Check sheet for the modelled part. Datum: model origin and axes. Units: mm. A direction names the side the tool comes from. Coordinates: 2 decimals unless noted, no trailing zeros. Loops run counter-clockwise (first coordinate to the right, second up) from the corner with the lowest first, then second, coordinate; pieces in that order, holes last.
```python
from build123d import *

# Parameters (mm, degrees)
F0_W     = 23.4204549342
F0_H     = 2.8636362404
F3_R     = 5
F5_W     = 35.1818175986
F5_H     = 36.409093067
F6_DEPTH = 64


# Not quite as in the source:
# - a fillet or chamfer that OpenCascade refuses, or shapes differently, is made with other operations: its cross-section is extruded or revolved along the edge and cut away or added


with BuildPart() as f1:
    # F0 (on Top) → F1 (revolve)
    with BuildSketch(Plane.XY):
        Polygon((-23.4204549342, 28.6363661289), (-26.4886375517, 28.6363661289), (-26.4886375517, -20.4545464367), (-23.4204549342, -20.4545464367), (-23.4204549342, -17.5909101963), align=None)
        with Locations((-11.7102274671, -19.0227283165)):
            Rectangle(F0_W, F0_H)
    revolve(axis=Axis((0, -19.0227283165, 0), (0, 1, 0)))

    # F3
    f3_edges = [f1.edges().sort_by_distance(p)[0] for p in [
        (26.488638, -20.454546, 0),
    ]]
    fillet(f3_edges, radius=F3_R)

    # F4: fillet of radius 5 on 1 edges, made by hand

    # F4_s1 → F4_t2 (revolve, cut)
    with BuildSketch(Plane.XY):
        with BuildLine():
            ThreePointArc((-26.4886375517, 28.6363661289), (-24.2575781097, 26.7941920001), (-23.4204549342, 24.0246330924))
            Line((-23.4204549342, 24.0246330924), (-23.4204549342, 28.6363661289))
            Line((-23.4204549342, 28.6363661289), (-26.4886375517, 28.6363661289))
        make_face()
    revolve(axis=Axis((0, 28.6363661289, 0), (0, 1, 0)), mode=Mode.SUBTRACT)

    # F5 (on offset) → F6 (cut)
    with BuildSketch(Plane.YZ.offset(-26.45)):
        with Locations((7.4659097008, -1.0227272287)):
            Rectangle(F5_W, F5_H)
    extrude(amount=-F6_DEPTH, mode=Mode.SUBTRACT)


solid = f1.part
```
1) Section check A-A on z = 0. Enter the section's corners in (x, y) (3 decimals), plus the area to 3 significant figures.
Answer sheet:
outline: (-26.489, -15.455) arc R5 ccw to (-21.489, -20.455) - (21.489, -20.455) arc R5 ccw to (26.489, -15.455) - (26.489, 28.636) arc R5 ccw to (23.42, 24.025) - (23.42, -17.591) - (-23.42, -17.591) - (-23.42, 24.025) arc R5 ccw to (-26.489, 28.636) - (-26.489, 25.057) - (-26.45, 25.057) - (-26.45, -10.125) - (-26.489, -10.125) - close
area: 415 mm2
2) Section check C-C on y = 10. Enter the section's corners in (x, z).
Answer sheet:
outline: (-26.45, -1.43) arc R26.49 ccw (long way) to (-26.45, 1.43) - close; hole circle Ø46.84 at (0, 0)
3) Depth check by flat-ended pin: pin 1 (6 mm diameter, centred on y = 14, z = 14, fed in from +X); pin 2 (8 mm diameter, centred on y = -9, z = 6.5, fed in from -X); pin 3 (10 mm diameter, centred on y = 19.5, z = -14.5, fed in from -X). Enter the tip coordinate at first touch or a pass-through.
Answer sheet:
pin 1: stops at x = 24.1
pin 2: stops at x = -26.37
pin 3: stops at x = -24.73
4) Set-up check for faces 1 (the cylindrical face through (5.077, 3.508, -22.864)), 2 (the flat face through (0, -20.455, 0)): record each of +Z, -Z, +X, -X, +Y, -Y from which the full face is reachable in a straight line by a thin tool's end or side.
Answer sheet:
face 1: +Y
face 2: +Z, -Z, +X, -X, -Y
5) Mould release check, pull along X, two halves, no side actions. Record for faces 3 (the cylindrical face through (-25.265, 6.282, 7.956)), 4 (the flat face through (-26.45, 7, 0)), 5 (the flat face through (0, -17.591, 0)): +X half, -X half, draft (parallel to the pull), parting line (faces both ways), or undercut.
Answer sheet:
face 3: parting line
face 4: -X half
face 5: undercut
6) Section check B-B on x = 0. Enter the section's corners in (y, z), plus the area to 3 significant figures.
Answer sheet:
outline: (-20.45, -21.49) arc R5 ccw to (-15.45, -26.49) - (28.64, -26.49) arc R5 ccw to (24.02, -23.42) - (-17.59, -23.42) - (-17.59, 23.42) - (24.02, 23.42) arc R5 ccw to (28.64, 26.49) - (-15.45, 26.49) arc R5 ccw to (-20.45, 21.49) - close
area: 417 mm2
7) Scan lines: line 1 (Z direction, x = 0, y = 8); line 2 (Y direction, x = 16, z = -9); line 3 (Z direction, x = -9, y = 14). Record each from-to range of solid material in increasing order.
Answer sheet:
line 1: z = -26.49 to -23.42, 23.42 to 26.49
line 2: y = -20.45 to -17.59
line 3: z = -24.91 to -21.62, 21.62 to 24.91
